Check sheet for the modelled part. Datum: model origin and axes. Units: mm. A direction names the side the tool comes from. Give positions to 0.01 mm unless a question says otherwise; leave off trailing zeros. Order: outer loops, then holes, each group sorted by start corner. A loop starts at its lowest first (then second) coordinate and runs counter-clockwise, first axis right, second up.
```python
from build123d import *

# Parameters (mm, degrees)
F0_W      = 58
F0_H      = 2
F1_DEPTH  = 42.5
F2_R      = 5
F3_R      = 2
F3_R_2    = 1
F4_DEPTH  = 4
F4_FACE_R = 1
F3_R_3    = 1.6
F5_DEPTH  = 2
F6_SIZE   = 0.5


with BuildPart() as f1:
    # F0 (on Front) → F1 (new body, symmetric)
    with BuildSketch(Plane.XZ):
        with Locations((0, 1)):
            Rectangle(F0_W, F0_H)
    extrude(amount=F1_DEPTH, both=True)

    # F2
    f2_edges = [f1.edges().sort_by_distance(p)[0] for p in [
        (-29, 42.5, 1),
        (29, 42.5, 1),
        (29, -42.5, 1),
        (-29, -42.5, 1),
    ]]
    fillet(f2_edges, radius=F2_R)

    # F3 (on face) → F4 (join)
    with BuildSketch(Plane(origin=(0, 0, 0), x_dir=(1, 0, 0), z_dir=(0, 0, -1))):
        with Locations((-24, -39.02)):
            Circle(F3_R)
        with Locations((-24, -39.02)):
            Circle(F3_R_2, mode=Mode.SUBTRACT)
        with Locations((-24, 18.9)):
            Circle(F3_R)
        with Locations((-24, 18.9)):
            Circle(F3_R_2, mode=Mode.SUBTRACT)
        with Locations((25, -39.02)):
            Circle(F3_R)
        with Locations((25, -39.02)):
            Circle(F3_R_2, mode=Mode.SUBTRACT)
        with Locations((25, 18.9)):
            Circle(F3_R)
        with Locations((25, 18.9)):
            Circle(F3_R_2, mode=Mode.SUBTRACT)
    extrude(amount=F4_DEPTH)

    # F4_face (on face) + F3 (on face) → F5 (cut, through all)
    with BuildSketch(Plane(origin=(-24, 39.02, 0), x_dir=(1, 0, 0), z_dir=(0, 0, -1))):
        Circle(F4_FACE_R)
        with Locations((0, 57.92)):
            Circle(F4_FACE_R)
        with Locations((49, 57.92)):
            Circle(F4_FACE_R)
        with Locations((49, 0)):
            Circle(F4_FACE_R)
    with BuildSketch(Plane(origin=(0, 0, 0), x_dir=(1, 0, 0), z_dir=(0, 0, -1))):
        with Locations((-19, -32)):
            Circle(F3_R_3)
        with Locations((20, -32)):
            Circle(F3_R_3)
        with Locations((-19, 31)):
            Circle(F3_R_3)
        with Locations((20, 31)):
            Circle(F3_R_3)
    extrude(amount=-F5_DEPTH, mode=Mode.SUBTRACT)

    # F6
    f6_edges = [f1.edges().sort_by_distance(p)[0] for p in [
        (0, 42.5, 2),
        (29, 0, 0),
    ]]
    chamfer(f6_edges, length=F6_SIZE)


solid = f1.part
```
(1) Cross-section at A-A on z = -2. Enter the section's corners in (x, y).
Response values:
outline: circle Ø4 at (-24, -18.9); circle Ø4 at (-24, 39.02); circle Ø4 at (25, -18.9); circle Ø4 at (25, 39.02); hole circle Ø2 at (-24, -18.9); hole circle Ø2 at (-24, 39.02); hole circle Ø2 at (25, -18.9); hole circle Ø2 at (25, 39.02)
(2) Cross-section at D-D on y = 9. Enter the section's corners in (x, z), then the cut area to 4 significant figures.
Response values:
outline: (-29, 0.5) - (-28.5, 0) - (28.5, 0) - (29, 0.5) - (29, 1.5) - (28.5, 2) - (-28.5, 2) - (-29, 1.5) - close
area: 115.5 mm2
(3) Set-up check for faces 4 (the face through (-24.434, 40.972, -1.972)), 5 (the face through (27.246, 40.819, 0.142)): record each of +Z, -Z, +X, -X, +Y, -Y from which the full face is reachable in a straight line by a thin tool's end or side.
Response values:
face 4: -Z
face 5: -Z, +X, +Y
(4) Material ranges on L1, parallel to X at y = 39.02, z = -1.95; L2, parallel to Y at x = -24, z = -2.7; L3, parallel to X at y = -31, z = 0.85, recorded low to high.
Response values:
L1: x = -26 to -25, -23 to -22, 23 to 24, 26 to 27
L2: y = -20.9 to -19.9, -17.9 to -16.9, 37.02 to 38.02, 40.02 to 41.02
L3: x = -29 to -20.6, -17.4 to 18.4, 21.6 to 29
(5) Gauge pin test, flat ends, axial feed: pin 1 Ø4 at (x, y) = (-19, -31) entering from -Z; pin 2 Ø4 at (x, y) = (20, 32) entering from +Z. Record the tip position at first contact, or that the pin passes through.
Response values:
pin 1: stops at z = 0
pin 2: stops at z = 2
(6) Cross-section at B-B on x = 20. Enter the section's corners in (y, z).
Response values:
outline: (-42.5, 0.5) - (-42, 0) - (-32.6, 0) - (-32.6, 2) - (-42, 2) - (-42.5, 1.5) - close; (-29.4, 0) - (30.4, 0) - (30.4, 2) - (-29.4, 2) - close; (33.6, 0) - (42, 0) - (42.5, 0.5) - (42.5, 1.5) - (42, 2) - (33.6, 2) - close
(7) Release check for a two-part mould opening along X. For faces 1 (the face through (18.73, 32.97, 0.99)), 2 (the face through (0, -1, 2)), 3 (the face through (-27.246, -40.819, 0.142)) record: released by +X, released by -X, zero draft, split by the parting line, or undercut.
Response values:
face 1: undercut
face 2: zero draft
face 3: released by -X
(8) Cross-section at C-C on y = -18.9. Enter the section's corners in (x, z), then the cut area to 4 significant figures.
Response values:
outline: (-29, 0.5) - (-28.5, 0) - (-26, 0) - (-26, -4) - (-25, -4) - (-25, 2) - (-28.5, 2) - (-29, 1.5) - close; (-23, -4) - (-22, -4) - (-22, 0) - (23, 0) - (23, -4) - (24, -4) - (24, 2) - (-23, 2) - close; (26, -4) - (27, -4) - (27, 0) - (28.5, 0) - (29, 0.5) - (29, 1.5) - (28.5, 2) - (26, 2) - close
area: 123.5 mm2
